from build123d import *

# Parameters (mm, degrees)
F0_R      = 11
F1_DEPTH  = 25
F3_R      = 1.525
F4_DEPTH  = 105.2
F5_DEPTH  = 11
F7_DEPTH  = 11
F0_R_2    = 7.5
F8_DEPTH  = 20
F9_DEPTH  = 5
F10_R     = 2
F11_DEPTH = 10
F13_DEPTH = 25.0010001
F14_DEPTH = 6
F15_DEPTH = 10
F16_R     = 3.25
F17_DEPTH = 25


# Not quite as in the source:
# - a feature names something its author has since deleted; it is built from what else it names


with BuildPart() as f1:
    # F0 (on Top) → F1 (new body)
    with BuildSketch(Plane.XY):
        with BuildLine():
            Line((90, -8), (0, -8))
            Line((0, -8), (0, -25))
            ThreePointArc((0, -25), (4.0455488499, -35.246950766), (14, -39.9666295471))
            Line((14, -39.9666295471), (14, -32.9160797831))
            ThreePointArc((14, -32.9160797831), (9, -27), (14, -21.0839202169))
            Line((14, -21.0839202169), (14, -14))
            Line((14, -14), (16, -14))
            Line((16, -14), (16, -21.0839202169))
            ThreePointArc((16, -21.0839202169), (19.582575695, -23.1270166538), (21, -27))
            ThreePointArc((21, -27), (19.582575695, -30.8729833462), (16, -32.9160797831))
            Line((16, -32.9160797831), (16, -40))
            Line((16, -40), (74, -40))
            Line((74, -40), (74, -32.9160797831))
            ThreePointArc((74, -32.9160797831), (69, -27), (74, -21.0839202169))
            Line((74, -21.0839202169), (74, -14))
            Line((74, -14), (76, -14))
            Line((76, -14), (76, -21.0839202169))
            ThreePointArc((76, -21.0839202169), (79.582575695, -23.1270166538), (81, -27))
            ThreePointArc((81, -27), (79.582575695, -30.8729833462), (76, -32.9160797831))
            Line((76, -32.9160797831), (76, -39.9666295471))
            ThreePointArc((76, -39.9666295471), (85.9544511501, -35.246950766), (90, -25))
            Line((90, -25), (90, -8))
        make_face()
        with Locations((45, -20.9553470761)):
            Circle(F0_R, mode=Mode.SUBTRACT)
        with BuildLine():
            Line((14, -14), (14, -21.0839202169))
            ThreePointArc((14, -21.0839202169), (15, -21), (16, -21.0839202169))
            Line((16, -21.0839202169), (16, -14))
            Line((16, -14), (14, -14))
        make_face()
        with BuildLine():
            ThreePointArc((74, -21.0839202169), (75, -21), (76, -21.0839202169))
            Line((76, -21.0839202169), (76, -14))
            Line((76, -14), (74, -14))
            Line((74, -14), (74, -21.0839202169))
        make_face()
    extrude(amount=F1_DEPTH)

    # F3 (on Right) → F4 (cut)
    with BuildSketch(Plane.YZ):
        with Locations((-36.9413755834, 11.0567829106)):
            Circle(F3_R)
        with Locations((-36.9413755834, 20.1872170437)):
            Circle(F3_R)
    extrude(amount=F4_DEPTH, mode=Mode.SUBTRACT)

    # F3 (on Right) → F5 (cut)
    with BuildSketch(Plane.YZ):
        with BuildLine():
            Line((-39.7998355329, 24.9966811389), (-39.7998355329, 6.4961747266))
            Line((-39.7998355329, 6.4961747266), (-39.6976853907, 6.4961747266))
            ThreePointArc((-39.6976853907, 6.4961747266), (-36.1621514848, 7.9606408207), (-34.6976853907, 11.4961747266))
            Line((-34.6976853907, 11.4961747266), (-34.6976853907, 19.9966811389))
            ThreePointArc((-34.6976853907, 19.9966811389), (-36.1621514848, 23.5322150448), (-39.6976853907, 24.9966811389))
            Line((-39.6976853907, 24.9966811389), (-39.7998355329, 24.9966811389))
        make_face()
        with Locations((-36.9413755834, 11.0567829106)):
            Circle(F3_R, mode=Mode.SUBTRACT)
        with Locations((-36.9413755834, 20.1872170437)):
            Circle(F3_R, mode=Mode.SUBTRACT)
    extrude(amount=F5_DEPTH, mode=Mode.SUBTRACT)

    # F6 (on offset) → F7 (cut)
    with BuildSketch(Plane.YZ.offset(90)):
        with BuildLine():
            Line((-39.7998355329, 24.9966811389), (-39.7998355329, 6.4961747266))
            Line((-39.7998355329, 6.4961747266), (-39.6976853907, 6.4961747266))
            ThreePointArc((-39.6976853907, 6.4961747266), (-36.1621514848, 7.9606408207), (-34.6976853907, 11.4961747266))
            Line((-34.6976853907, 11.4961747266), (-34.6976853907, 19.9966811389))
            ThreePointArc((-34.6976853907, 19.9966811389), (-36.1621514848, 23.5322150448), (-39.6976853907, 24.9966811389))
            Line((-39.6976853907, 24.9966811389), (-39.7998355329, 24.9966811389))
        make_face()
    extrude(amount=-F7_DEPTH, mode=Mode.SUBTRACT)

    # F0 (on Top) → F8 (join)
    with BuildSketch(Plane.XY):
        with Locations((45, -20.9553470761)):
            Circle(F0_R)
        with Locations((45, -20.9553470761)):
            Circle(F0_R_2, mode=Mode.SUBTRACT)
    extrude(amount=F8_DEPTH)

    # F0 (on Top) → F9 (cut)
    with BuildSketch(Plane.XY):
        with Locations((45, -20.9553470761)):
            Circle(F0_R)
        with Locations((45, -20.9553470761)):
            Circle(F0_R_2, mode=Mode.SUBTRACT)
    extrude(amount=F9_DEPTH, mode=Mode.SUBTRACT)

    # F10 (on face) → F11 (cut)
    with BuildSketch(Plane(origin=(0, -8, 0), x_dir=(-1, 0, 0), z_dir=(0, 1, 0))):
        with Locations((-28.83, 18.75)):
            Circle(F10_R)
        with Locations((-61.17, 18.75)):
            Circle(F10_R)
    extrude(amount=-F11_DEPTH, mode=Mode.SUBTRACT)

    # F12 (on face) → F13 (cut, through all)
    with BuildSketch(Plane.XY.offset(25)):
        with BuildLine():
            Line((45, -40), (45, -34.6395410597))
            Line((45, -34.6395410597), (25.387, -34.6395410597))
            ThreePointArc((25.387, -34.6395410597), (23.6991374304, -35.338675856), (23, -37.0265373344))
            Line((23, -37.0265373344), (23, -40))
            Line((23, -40), (45, -40))
        make_face()
        with BuildLine():
            ThreePointArc((67, -36.7889047916), (66.2265029782, -35.2566531011), (64.6248583192, -34.6395410597))
            Line((64.6248583192, -34.6395410597), (45, -34.6395410597))
            Line((45, -34.6395410597), (45, -40))
            Line((45, -40), (67, -40))
            Line((67, -40), (67, -36.7889047916))
        make_face()
    extrude(amount=-F13_DEPTH, mode=Mode.SUBTRACT)

    # F0 (on Top) → F14 (cut)
    with BuildSketch(Plane.XY):
        with BuildLine():
            Line((90, -8), (0, -8))
            Line((0, -8), (0, -25))
            ThreePointArc((0, -25), (4.0455488499, -35.246950766), (14, -39.9666295471))
            Line((14, -39.9666295471), (14, -32.9160797831))
            ThreePointArc((14, -32.9160797831), (9, -27), (14, -21.0839202169))
            Line((14, -21.0839202169), (14, -14))
            Line((14, -14), (16, -14))
            Line((16, -14), (16, -21.0839202169))
            ThreePointArc((16, -21.0839202169), (19.582575695, -23.1270166538), (21, -27))
            ThreePointArc((21, -27), (19.582575695, -30.8729833462), (16, -32.9160797831))
            Line((16, -32.9160797831), (16, -40))
            Line((16, -40), (74, -40))
            Line((74, -40), (74, -32.9160797831))
            ThreePointArc((74, -32.9160797831), (69, -27), (74, -21.0839202169))
            Line((74, -21.0839202169), (74, -14))
            Line((74, -14), (76, -14))
            Line((76, -14), (76, -21.0839202169))
            ThreePointArc((76, -21.0839202169), (79.582575695, -23.1270166538), (81, -27))
            ThreePointArc((81, -27), (79.582575695, -30.8729833462), (76, -32.9160797831))
            Line((76, -32.9160797831), (76, -39.9666295471))
            ThreePointArc((76, -39.9666295471), (85.9544511501, -35.246950766), (90, -25))
            Line((90, -25), (90, -8))
        make_face()
        with Locations((45, -20.9553470761)):
            Circle(F0_R, mode=Mode.SUBTRACT)
        with BuildLine():
            Line((14, -14), (14, -21.0839202169))
            ThreePointArc((14, -21.0839202169), (15, -21), (16, -21.0839202169))
            Line((16, -21.0839202169), (16, -14))
            Line((16, -14), (14, -14))
        make_face()
        with BuildLine():
            ThreePointArc((74, -21.0839202169), (75, -21), (76, -21.0839202169))
            Line((76, -21.0839202169), (76, -14))
            Line((76, -14), (74, -14))
            Line((74, -14), (74, -21.0839202169))
        make_face()
        with Locations((45, -20.9553470761)):
            Circle(F0_R)
        with Locations((45, -20.9553470761)):
            Circle(F0_R_2, mode=Mode.SUBTRACT)
    extrude(amount=F14_DEPTH, mode=Mode.SUBTRACT)

    # F0 (on Top) → F15 (cut)
    with BuildSketch(Plane.XY):
        with Locations((45, -20.9553470761)):
            Circle(F0_R)
        with Locations((45, -20.9553470761)):
            Circle(F0_R_2, mode=Mode.SUBTRACT)
    extrude(amount=F15_DEPTH, mode=Mode.SUBTRACT)

    # F16 (on face) → F17 (cut)
    with BuildSketch(Plane.XZ.offset(40)):
        with Locations((28.83, 18.75)):
            Circle(F16_R)
        with Locations((61.17, 18.75)):
            Circle(F16_R)
    extrude(amount=-F17_DEPTH, mode=Mode.SUBTRACT)


solid = f1.part
Verification items for the finished model (mm, model axes). A direction names the side the tool comes from. Coordinates: 2 decimals unless noted, no trailing zeros. Loops run counter-clockwise (first coordinate to the right, second up) from the corner with the lowest first, then second, coordinate; pieces in that order, holes last. Notation, with made-up numbers: (-33, 35) -> (-8, 35) arc R29 ccw to (-8, 55) -> close; hole circle Ø2 at (31.5, 5.25). An arc over 180 degrees is marked (long way). Answer as CSV lines item,"result".
1) Thickness scan on L1, parallel to X at y = -39, z = 7.25; L2, parallel to X at y = -13, z = 19.25; L3, parallel to X at y = -28, z = 20.75. Record the ranges inside material, lowest first. Write a range as from..to.
Found:
L1,"x = 11..14, 16..23, 67..74, 76..79"
L2,"x = 0..26.89, 30.77..59.23, 63.11..90"
L3,"x = 0.3..9.08, 20.92..26.27, 31.39..36.55, 53.45..58.61, 63.73..69.08, 80.92..89.7"
2) Cross-section at D-D, the plane z = 14. Record the cut outline in (x, y), then the cut area to 3 significant figures.
Found:
outline,"(0, -25) arc R15 ccw to (3.56, -34.7) -> (11, -34.7) -> (11, -39.46) arc R15 ccw to (14, -39.97) -> (14, -32.92) arc R6 cw (long way) to (16, -32.92) -> (16, -40) -> (23, -40) -> (23, -37.03) arc R2.39 cw to (25.39, -34.64) -> (64.62, -34.64) arc R2.39 cw to (67, -36.79) -> (67, -40) -> (74, -40) -> (74, -32.92) arc R6 cw (long way) to (76, -32.92) -> (76, -39.97) arc R15 ccw to (79, -39.46) -> (79, -34.7) -> (86.44, -34.7) arc R15 ccw to (90, -25) -> (90, -8) -> (0, -8) -> close; hole circle Ø15 at (45, -20.96)"
area,"2,080 mm2"
3) Cross-section at B-B, the plane y = -19. Record the cut outline in (x, z).
Found:
outline,"(0, 6) -> (34.18, 6) -> (34.18, 10) -> (37.76, 10) -> (37.76, 20) -> (34.18, 20) -> (34.18, 25) -> (0, 25) -> close; (52.24, 10) -> (55.82, 10) -> (55.82, 6) -> (90, 6) -> (90, 25) -> (55.82, 25) -> (55.82, 20) -> (52.24, 20) -> close; hole circle Ø6.5 at (28.83, 18.75); hole circle Ø6.5 at (61.17, 18.75)"
4) Cross-section at A-A, the plane y = -26. Record the cut outline in (x, z), then the cut area to 3 significant figures.
Found:
outline,"(0.03, 6) -> (9.08, 6) -> (9.08, 25) -> (0.03, 25) -> close; (20.92, 6) -> (35.22, 6) -> (35.22, 10) -> (39.45, 10) -> (39.45, 20) -> (35.22, 20) -> (35.22, 25) -> (20.92, 25) -> close; (50.55, 10) -> (54.78, 10) -> (54.78, 6) -> (69.08, 6) -> (69.08, 25) -> (54.78, 25) -> (54.78, 20) -> (50.55, 20) -> close; (80.92, 6) -> (89.97, 6) -> (89.97, 25) -> (80.92, 25) -> close; hole circle Ø6.5 at (28.83, 18.75); hole circle Ø6.5 at (61.17, 18.75)"
area,"906 mm2"
5) Depth check by flat-ended pin: pin 1 (9.5 mm diameter, centred on x = 38.5, z = 11, fed in from -Y); pin 2 (12 mm diameter, centred on x = 45, y = -20.96, fed in from +Z); pin 3 (11 mm diameter, centred on x = 43.5, y = -17.5, fed in from -Z); pin 4 (5 mm diameter, centred on y = -30.5, z = 23, fed in from -X). Enter the tip coordinate at first touch or a pass-through.
Found:
pin 1,"stops at y = -34.64"
pin 2,"passes through"
pin 3,"stops at z = 10"
pin 4,"stops at x = 0.3"
6) Release check for a two-part mould opening along Z. For faces 1 (the flat face through (23, -38, 16)), 2 (the flat face through (42, -28, 10)), 3 (the cylindrical face through (30.828, -11.451, 18.838)) record: +Z half, -Z half, draft (parallel to the pull), parting line (faces both ways), or undercut.
Found:
face 1,"draft"
face 2,"-Z half"
face 3,"undercut"
7) Cross-section at C-C, the plane x = 45. Record the cut outline in (y, z).
Found:
outline,"(-34.64, 6) -> (-31.96, 6) -> (-31.96, 10) -> (-28.46, 10) -> (-28.46, 20) -> (-31.96, 20) -> (-31.96, 25) -> (-34.64, 25) -> close; (-13.46, 10) -> (-9.96, 10) -> (-9.96, 6) -> (-8, 6) -> (-8, 25) -> (-9.96, 25) -> (-9.96, 20) -> (-13.46, 20) -> close"
8) Tool access check on faces 4 (the cylindrical face through (50.1, -30.7, 22.5)), 5 (the flat face through (63, -15, 20)), 6 (the flat face through (79, -38, 16)), 7 (the flat face through (7, -34.698, 16)). Record the directions out of +Z, -Z, +X, -X, +Y, -Y that give a thin tool (end or side, any length) a straight path to the whole face; none if there is none.
Found:
face 4,"+Z"
face 5,"-Y"
face 6,"+X, -Y"
face 7,"-X, -Y"
